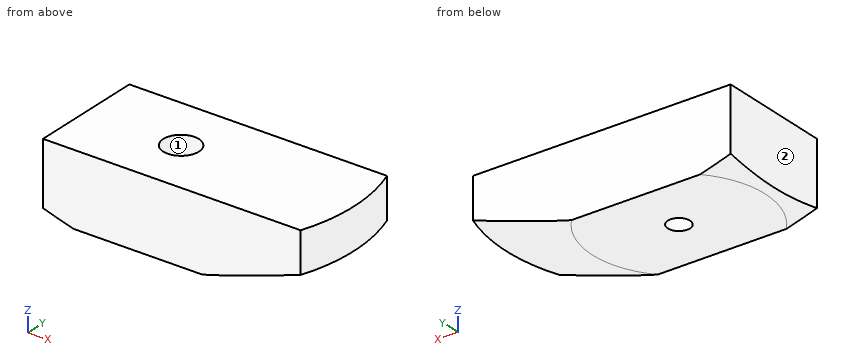
```python
from build123d import *

# Parameters (mm, degrees)
SKETCH1_R           = 38.1
BOSS_EXTRUDE1_DEPTH = 15.875
SKETCH2_R           = 3.937
CUT_EXTRUDE1_DEPTH  = 5.715
SKETCH3_R           = 2.450575626
CUT_EXTRUDE2_DEPTH  = 55.831064188
CHAMFER1_SIZE       = 19.05
CHAMFER1_SIZE2      = 6.933632963
CUT_EXTRUDE3_DEPTH  = 57.171484091


with BuildPart() as part:
    # Sketch1 → Boss-Extrude1 (new body)
    with BuildSketch(Plane.XY):
        Circle(SKETCH1_R)
    extrude(amount=BOSS_EXTRUDE1_DEPTH)

    # Sketch2 → Cut-Extrude1 (cut)
    with BuildSketch(Plane.XY.offset(15.875)):
        Circle(SKETCH2_R)
    extrude(amount=-CUT_EXTRUDE1_DEPTH, mode=Mode.SUBTRACT)

    # Sketch3 → Cut-Extrude2 (cut, through all)
    with BuildSketch(Plane.XY.offset(10.16)):
        Circle(SKETCH3_R)
    extrude(amount=-CUT_EXTRUDE2_DEPTH, mode=Mode.SUBTRACT)

    # Chamfer1
    chamfer1_edges = [part.edges().sort_by_distance(p)[0] for p in [
        (-38.1, 0, 0),
    ]]
    chamfer1_side = [part.faces().sort_by_distance(p)[0] for p in [
        (-37.022369265, 0, 0),
    ]]
    chamfer(chamfer1_edges, length=CHAMFER1_SIZE, length2=CHAMFER1_SIZE2, reference=chamfer1_side[0])

    # Sketch4 → Cut-Extrude3 (cut, through all)
    with BuildSketch(Plane.XY.offset(15.875)):
        with BuildLine():
            ThreePointArc((35.921024484, 12.7), (-38.1, 0), (35.921024484, -12.7))
            Line((35.921024484, -12.7), (-20.955, -12.7))
            Line((-20.955, -12.7), (-20.955, 12.7))
            Line((-20.955, 12.7), (35.921024484, 12.7))
        make_face()
    extrude(amount=-CUT_EXTRUDE3_DEPTH, mode=Mode.SUBTRACT)


solid = part.part
```
The model under review builds one solid part; all positions refer to its coordinate system, in mm. Face numbers are marked on the shaded views. A direction names the side the tool comes from. Round coordinates to 2 decimals unless told otherwise and drop trailing zeros. Loops run counter-clockwise (first coordinate to the right, second up) from the corner with the lowest first, then second, coordinate; pieces in that order, holes last. Notation, with made-up numbers: (2, 10.5) - (22, 10.5) arc R30 cw to (22, 36.5) - close; hole circle Ø9 at (24, 73). An arc over 180 degrees is marked (long way). Use a Markdown table: item, result. Add a question column.
Q1. Insertion check: pin 1 Ø4.5 at (x, y) = (0, 0) entering from +Z; pin 2 Ø1 at (x, y) = (3, 7.5) entering from -Z; pin 3 Ø2.5 at (x, y) = (1.5, 2) entering from +Z. Each pin has a flat end and moves straight along its axis. Give the tip position at first contact, or say it passes through.
Q2. Add section C-C (z = 8). State the section outline as (x, y) points (3 decimals), plus the area to 3 significant figures.
Q3. Add section B-B (x = 0). State the section outline as (y, z) points (3 decimals), plus the area to 3 significant figures.
Q4. For probe 1 along Y at (x, z) = (0, 9.5); probe 2 along Y at (x, z) = (0, 12.45); probe 3 along X at (y, z) = (-2.25, 11) (1 decimal), list the stretches that pass through material, from the lowest coordinate up.
Q5. Add section A-A (y = 0). State the section outline as (x, z) points (3 decimals), plus the area to 3 significant figures.
Q6. Machinability: for the marked faces 1 and 2, which of the approach directions +Z, -Z, +X, -X, +Y, -Y give a long, thin tool a straight path to every point of the face, cutting with its end or side? Answer none if there is none.
Q7. Add section D-D (z = 10.75). State the section outline as (x, y) points (3 decimals), plus the area to 3 significant figures.
Worked answers:
| question | item | result |
|---|---|---|
| 1 | pin 1 | through |
| 1 | pin 2 | z = 0 |
| 1 | pin 3 | z = 10.16 |
| 2 | outline | (-20.955, -12.7) - (35.921, -12.7) arc R38.1 ccw to (35.921, 12.7) - (-20.955, 12.7) - close; hole circle Ø4.901 at (0, 0) |
| 2 | area | 1,460 mm² |
| 3 | outline | (-12.7, 0) - (-2.451, 0) - (-2.451, 10.16) - (-3.937, 10.16) - (-3.937, 15.875) - (-12.7, 15.875) - close; (2.451, 0) - (12.7, 0) - (12.7, 15.875) - (3.937, 15.875) - (3.937, 10.16) - (2.451, 10.16) - close |
| 3 | area | 308 mm² |
| 4 | probe 1 | -12.7 to -2.45, 2.45 to 12.7 |
| 4 | probe 2 | -12.7 to -3.94, 3.94 to 12.7 |
| 4 | probe 3 | -21 to -3.2, 3.2 to 38 |
| 5 | outline | (-20.955, 0.693) - (-19.05, 0) - (-2.451, 0) - (-2.451, 10.16) - (-3.937, 10.16) - (-3.937, 15.875) - (-20.955, 15.875) - close; (2.451, 0) - (19.05, 0) - (38.1, 6.934) - (38.1, 15.875) - (3.937, 15.875) - (3.937, 10.16) - (2.451, 10.16) - close |
| 5 | area | 776 mm² |
| 6 | face 1 | +Z |
| 6 | face 2 | +Z, -Z, -X, +Y, -Y |
| 7 | outline | (-20.955, -12.7) - (35.921, -12.7) arc R38.1 ccw to (35.921, 12.7) - (-20.955, 12.7) - close; hole circle Ø7.874 at (0, 0) |
| 7 | area | 1,430 mm² |
